The model under review builds one solid part; all positions refer to its coordinate system, in mm. Face numbers are marked on the shaded views. A direction names the side the tool comes from. Give positions to 0.01 mm unless a question says otherwise; leave off trailing zeros. Loops run counter-clockwise (first coordinate to the right, second up) from the corner with the lowest first, then second, coordinate; pieces in that order, holes last. Notation, with made-up numbers: M 89.25,23 L 134.25,23 A16 cw 134.25,37 Z; hole C 19,72.5 d3. An arc over 180 degrees is marked long. Return JSON: item names as keys, results as strings.
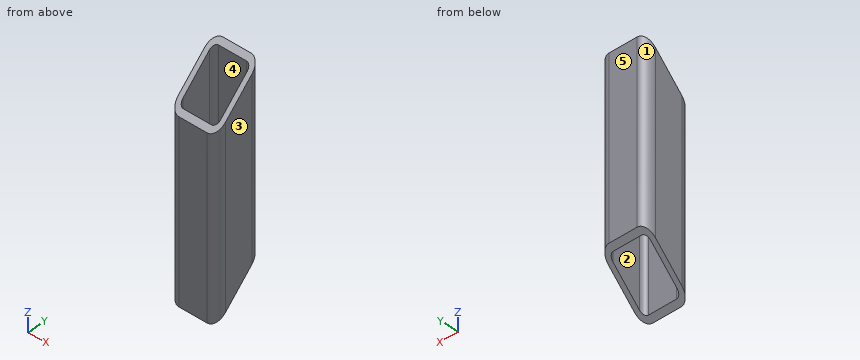
Autodesk Inventor part; units mm, degrees
ref_plane "Start Plane" through (0, 0, 0) normal (0, 0, 1) x (1, 0, 0)
ref_plane "End Plane" through (0, 0, 94.7523) normal (0, 0, 1) x (1, 0, 0)
ref_plane "YZ Plane" through (0, 0, 0) normal (1, 0, 0) x (0, 1, 0)
ref_plane "Start Plane" through (0, 0, 0) normal (0, 0, 1) x (1, 0, 0)
ref_plane "End Plane" through (0, 0, 94.7523) normal (0, 0, 1) x (1, 0, 0)
sketch "Sketch" plane through (0, 0, 0) normal (0, 0, 1) x (1, 0, 0)
  line L0 (-10, -6) -> (-10, 6)
  line L1 (-6, 10) -> (6, 10)
  line L2 (10, 6) -> (10, -6)
  line L3 (6, -10) -> (-6, -10)
  arc A0 (-10, -6) -> (-6, -10) centre (-6, -6) ccw
  arc A1 (10, 6) -> (6, 10) centre (6, 6) ccw
  arc A2 (-6, 10) -> (-10, 6) centre (-6, 6) ccw
  arc A3 (6, -10) -> (10, -6) centre (6, -6) ccw
  arc A4 (-6, 8) -> (-8, 6) centre (-6, 6) ccw
  line L4 (-6, 8) -> (6, 8)
  arc A5 (8, 6) -> (6, 8) centre (6, 6) ccw
  line L5 (8, 6) -> (8, -6)
  arc A6 (6, -8) -> (8, -6) centre (6, -6) ccw
  line L6 (6, -8) -> (-6, -8)
  arc A7 (-8, -6) -> (-6, -8) centre (-6, -6) ccw
  line L7 (-8, -6) -> (-8, 6)
  line L8 (0, 15.1598) -> (0, -15.1598) construction
  line L9 (-15.1598, 0) -> (15.1598, 0) construction
  dimension "d7" = 4
  dimension "d9" = 20
  dimension "d11" = 20
  dimension "d12" = 2
  dimension "d15" = 10
  dimension "d16" = 10
extrude "Body" add sketch "Sketch" along normal up to surface (94.7523 mm away) from surface at 0
sketch "Sketch3" plane through (0, 0, 0) normal (0, 0, 1) x (1, 0, 0)
  line L0 (0, 0) -> (10, 0)
ref_plane "Work Plane3" through (0, 0, 0) normal (0, -1, 0) x (1, 0, 0)
sketch "Sketch5" plane through (10, -6, 94.7523) normal (1, 0, 0) x (0, 0, -1)
  line L0 (0, 12) -> (0, 16)
  line L1 (0, 16) -> (20, -4)
  line L2 (94.7523, -4) -> (0, -4)
  line L3 (94.7523, 16) -> (0, 16)
  line L4 (74.7523, 16) -> (94.7523, -4)
  line L5 (0, 12) -> (0, 0)
  line L6 (0, -4) -> (0, 0)
  line L7 (94.7523, -4) -> (0, -4)
  line L8 (94.7523, 12) -> (94.7523, 0)
  line L9 (94.7523, 12) -> (94.7523, 16)
  line L10 (94.7523, -4) -> (94.7523, 0)
  point P0 (94.7523, 6)
  point P1 (84.7523, 6)
  dimension "d19" = 45
extrude "Extrusion2" cut sketch "Sketch5" against normal through all contours L0 L1 L2 L6 L5 | L3 L9 L8 L10 L4
sketch "Sketch4" plane through (0, 0, 0) normal (0, -1, 0) x (1, 0, 0)
  line L0 (-2, 0) -> (12, 0)
  line L1 (-2, 94.7523) -> (12, 94.7523)
  dimension "d18" = 94.7523
equation "\"d7\" = G_IR"
equation "\"d9\" = G_W"
equation "\"d11\" = G_H"
equation "\"d12\" = G_T"
equation "\"d15\" = 0.5 * d9"
equation "\"d16\" = 0.5 * d11"
equation "\"d3\" = G_L"
equation "\"G_W\" = 20"
equation "\"G_H\" = 20"
equation "\"G_T\" = 2"
equation "\"G_IR\" = 4"
equation "\"G_L\" = d18"
equation "\"G_OFFSET_START\" = 0"
equation "\"G_OFFSET_END\" = 0"
equation "\"d14\" = G_OFFSET_END + B_L"
equation "\"B_L\" = 94.75231"
properties part number "ISO 10799-2 - 20x20x2 - 94,75" material "Steel, Mild"
1) Consider section C-C on y = 4.5. Write out the cut boundary in (x, z), then the cut area to 3 significant figures.
From the geometry:
{"outline": "M -10,14.5 L -8,14.5 L -8,89.25 L -10,89.25 Z; M 8,14.5 L 10,14.5 L 10,89.25 L 8,89.25 Z", "area": "299 mm²"}
2) Wall thickness on L1, parallel to X at y = 4.5, z = 32; L2, parallel to Y at x = 2, z = 16: over which ranges is each line inside the solid? List them lowest first. Write a range as from..to.
From the geometry:
{"L1": "-10..-8, 8..10", "L2": "-10..-8"}
3) Consider section B-B on z = 48.5. Write out the cut boundary in (x, y).
From the geometry:
{"outline": "M -10,-6 A4 ccw -6,-10 L 6,-10 A4 ccw 10,-6 L 10,6 A4 ccw 6,10 L -6,10 A4 ccw -10,6 Z; hole M -8,-6 A2 ccw -6,-8 L 6,-8 A2 ccw 8,-6 L 8,6 A2 ccw 6,8 L -6,8 A2 ccw -8,6 Z"}
4) The part is to be moulded in two halves that separate along Y. For the marked faces 1, 2 and 3, say which applies: released by +Y, released by -Y, zero draft, split by the parting line, or undercut.
From the geometry:
{"face 1": "released by +Y", "face 2": "undercut", "face 3": "zero draft"}
5) Tool access review of the marked faces 4 and 5: name each direction out of +Z, -Z, +X, -X, +Y, -Y from which nothing blocks a thin tool from reaching the whole face with its end or side.
From the geometry:
{"face 4": "+Z, -Z", "face 5": "+Z, -Z, +X, -X, +Y"}
6) Consider section D-D on z = 89.5. Write out the cut boundary in (x, y), then the cut area to 3 significant figures.
From the geometry:
{"outline": "M -10,4.75 L -8,4.75 L -8,6 A2 cw -6,8 L 6,8 A2 cw 8,6 L 8,4.75 L 10,4.75 L 10,6 A4 ccw 6,10 L -6,10 A4 ccw -10,6 Z", "area": "47.9 mm²"}
7) Insertion check: pin 1 (12 mm diameter, centred on x = 1.5, y = 0, fed in from -Z); pin 2 (2 mm diameter, centred on x = -7.5, y = 0, fed in from +Z); pin 3 (4 mm diameter, centred on x = -1.5, y = -6.5, fed in from -Z). Each pin has a flat end and moves straight along its axis. Give the tip position at first contact, or say it passes through.
From the geometry:
{"pin 1": "through", "pin 2": "z = 85.62", "pin 3": "z = 1.5"}
8) Consider section A-A on x = -2. Write out the cut boundary in (y, z).
From the geometry:
{"outline": "M -10,0 L -8,2 L -8,76.75 L -10,74.75 Z; M 8,18 L 10,20 L 10,94.75 L 8,92.75 Z"}
